Source: CAD feature listing. Evaluate the final solid. Frame: model axes, mm. A direction names the side the tool comes from. Give positions to 0.01 mm unless a question says otherwise; leave off trailing zeros. Loops run counter-clockwise (first coordinate to the right, second up) from the corner with the lowest first, then second, coordinate; pieces in that order, holes last.
```python
from build123d import *

# Parameters (mm, degrees)
F1_DEPTH  = 31.75
F2_R      = 6.35
F3_DEPTH  = 31.75
F5_DEPTH  = 31.75
F7_DEPTH  = 19.05
F8_DEPTH  = 6.35
F9_W      = 12.7
F9_H      = 12.7
F10_DEPTH = 31.75
F11_W     = 12.7
F11_H     = 12.7
F12_DEPTH = 19.05
F14_DEPTH = 12.7
F15_W     = 12.7
F15_H     = 12.7
F16_DEPTH = 12.7
F18_DEPTH = 12.7
F19_R     = 1.5875
F20_DEPTH = 12.7
F22_DEPTH = 6.35


# Not quite as in the source:
# - a feature names something its author has since deleted; it is built from what else it names


with BuildPart() as f1:
    # F0 (on Front) → F1 (new body)
    with BuildSketch(Plane.XZ):
        Polygon((-9.6981803781, 6.35), (-22.3981803781, 6.35), (-22.3981803781, 0), (28.4018196219, 0), (28.4018196219, 6.35), (15.7018196219, 6.35), (15.7018196219, 57.15), (-9.6981803781, 57.15), align=None)
    extrude(amount=F1_DEPTH)

    # F2 (on face) → F3 (cut)
    with BuildSketch(Plane.XZ.offset(31.75)):
        with Locations((3.0018196219, 44.45)):
            Circle(F2_R)
    extrude(amount=-F3_DEPTH, mode=Mode.SUBTRACT)

    # F4 (on face) → F5 (cut)
    with BuildSketch(Plane.XZ.offset(31.75)):
        with BuildLine():
            ThreePointArc((-9.6981803781, 44.45), (-5.9784365163, 53.4302561039), (3.0018195733, 57.15))
            Line((3.0018195733, 57.15), (-9.6981803781, 57.15))
            Line((-9.6981803781, 57.15), (-9.6981803781, 44.45))
        make_face()
        with BuildLine():
            ThreePointArc((3.0018195733, 57.15), (11.9820757258, 53.4302561383), (15.7018196219, 44.45))
            Line((15.7018196219, 44.45), (15.7018196219, 57.15))
            Line((15.7018196219, 57.15), (3.0018195733, 57.15))
        make_face()
    extrude(amount=-F5_DEPTH, mode=Mode.SUBTRACT)

    # F6 (on face) → F7 (cut)
    with BuildSketch(Plane.XZ.offset(31.75)):
        with BuildLine():
            Line((15.7018196219, 6.35), (15.7018196219, 44.45))
            ThreePointArc((15.7018196219, 44.45), (3.0018196219, 31.75), (-9.6981803781, 44.45))
            Line((-9.6981803781, 44.45), (-9.6981803781, 6.35))
            Line((-9.6981803781, 6.35), (15.7018196219, 6.35))
        make_face()
    extrude(amount=-F7_DEPTH, mode=Mode.SUBTRACT)

    # F8 (cut): a face of the model
    f8_faces = [f1.faces().sort_by_distance(p)[0] for p in [
        (15.3426093771, -31.75, 44.45),
    ]]
    extrude(f8_faces, amount=-F8_DEPTH, mode=Mode.SUBTRACT)

    # F9 (on face) → F10 (join)
    with BuildSketch(Plane.XZ.offset(31.75)):
        with Locations((-16.0481803781, 12.7)):
            Rectangle(F9_W, F9_H)
    extrude(amount=-F10_DEPTH)

    # F11 (on face) → F12 (cut)
    with BuildSketch(Plane.XZ.offset(31.75)):
        with Locations((-16.0481803781, 12.7)):
            Rectangle(F11_W, F11_H)
    extrude(amount=-F12_DEPTH, mode=Mode.SUBTRACT)

    # F13 (on face) → F14 (cut)
    with BuildSketch(Plane.XZ.offset(12.7)):
        with BuildLine():
            Line((-22.3981803781, 19.05), (-22.3981803781, 6.35))
            ThreePointArc((-22.3981803781, 6.35), (-13.417924257, 10.0697438789), (-9.6981803781, 19.05))
            Line((-9.6981803781, 19.05), (-22.3981803781, 19.05))
        make_face()
    extrude(amount=-F14_DEPTH, mode=Mode.SUBTRACT)

    # F15 (on face) → F16 (join)
    with BuildSketch(Plane.XZ.offset(12.7)):
        with Locations((22.0518196219, 12.7)):
            Rectangle(F15_W, F15_H)
    extrude(amount=-F16_DEPTH)

    # F17 (on face) → F18 (cut)
    with BuildSketch(Plane.XZ.offset(12.7)):
        with BuildLine():
            Line((28.4018196219, 19.05), (15.7018196219, 19.05))
            ThreePointArc((15.7018196219, 19.05), (19.4215635009, 10.0697438789), (28.4018196219, 6.35))
            Line((28.4018196219, 6.35), (28.4018196219, 19.05))
        make_face()
    extrude(amount=-F18_DEPTH, mode=Mode.SUBTRACT)

    # F19 (on Top) → F20 (cut)
    with BuildSketch(Plane.XY):
        with Locations((-12.8731803781, -22.225)):
            Circle(F19_R)
        with Locations((18.8768196219, -22.225)):
            Circle(F19_R)
    extrude(amount=-F20_DEPTH, mode=Mode.SUBTRACT)

    # F21 (on face) → F22 (cut)
    with BuildSketch(Plane.XY.offset(6.35)):
        with BuildLine():
            ThreePointArc((-9.6981803781, -31.75), (-18.6784364991, -28.0302561211), (-22.3981803781, -19.05))
            Line((-22.3981803781, -19.05), (-22.3981803781, -31.75))
            Line((-22.3981803781, -31.75), (-9.6981803781, -31.75))
        make_face()
        with BuildLine():
            ThreePointArc((28.4018196219, -19.05), (24.682075743, -28.0302561211), (15.7018196219, -31.75))
            Line((15.7018196219, -31.75), (28.4018196219, -31.75))
            Line((28.4018196219, -31.75), (28.4018196219, -19.05))
        make_face()
    extrude(amount=-F22_DEPTH, mode=Mode.SUBTRACT)


solid = f1.part
```
(1) Reachability of faces 5 (the flat face through (0, -25.4, 50.3)), 6 (the flat face through (15.702, -6, 32)), 7 (the flat face through (-9.698, -6, 32)) from +Z, -Z, +X, -X, +Y, -Y: full face, straight path, thin tool, end or side. Return the list, or none.
A:
face 5: +Z, +X, -X, -Y
face 6: +Z, +X, +Y, -Y
face 7: +Z, -X, +Y, -Y
(2) Mould query, pull axis Z, two halves, no side actions, for faces 1 (the flat face through (3, -16, 0)), 2 (the flat face through (3, -22, 6.35)), 3 (the cylindrical face through (19.32, -6.44, 10.17)), 4 (the cylindrical face through (24.78, -27.93, 3.22)). Classes: pulls with the +Z half, pulls with the -Z half, needs draft (parallel to the pull), parting line crosses it, or undercut.
A:
face 1: pulls with the -Z half
face 2: undercut
face 3: pulls with the +Z half
face 4: needs draft
(3) Section D-D, the plane x = 13.5. Return the cut outline in (y, z).
A:
outline: (-31.75, 0) - (0, 0) - (0, 51.6) - (-25.4, 51.6) - (-25.4, 37.3) - (-12.7, 37.3) - (-12.7, 6.35) - (-31.75, 6.35) - close
(4) Ray query, line 1 along Z through (x, y) = (3, -25); line 2 along Z through (x, y) = (3, -5.5); line 3 along Z through (x, y) = (-17.5, -27). Return the intervals inside material, ascending.
A:
line 1: z = 0 to 6.35, 31.75 to 38.1, 50.8 to 57.15
line 2: z = 0 to 38.1, 50.8 to 57.15
line 3: z = 0 to 6.35
(5) First-contact query: pin 1 (5 mm diameter, centred on x = 17, y = -26, fed in from +Z); pin 2 (12.5 mm diameter, centred on x = 0, z = 50.5, fed in from -Y); pin 3 (10 mm diameter, centred on y = -7, z = 26, fed in from +X); pin 4 (10 mm diameter, centred on x = 3, z = 44.45, fed in from +Y). Flat tips, straight axial feed; report the tip coordinate or a pass-through.
A:
pin 1: stops at z = 49.68
pin 2: stops at y = -25.4
pin 3: stops at x = 15.7
pin 4: passes through
(6) Section B-B, the plane y = -9.5. Return the cut outline in (x, z), then the cut area to 3 significant figures.
A:
outline: (-22.4, 0) - (28.4, 0) - (28.4, 6.35) arc R12.7 cw to (15.7, 19.05) - (15.7, 44.45) arc R12.7 ccw to (-9.7, 44.45) - (-9.7, 19.05) arc R12.7 cw to (-22.4, 6.35) - close; hole circle Ø12.7 at (3, 44.45)
area: 1,490 mm2
(7) Section A-A, the plane y = -17.5. Return the cut outline in (x, z), then the cut area to 3 significant figures.
A:
outline: (-22.4, 0) - (28.4, 0) - (28.4, 6.35) - (-22.4, 6.35) - close; circle Ø25.4 at (3, 44.45); hole circle Ø12.7 at (3, 44.45)
area: 703 mm2
